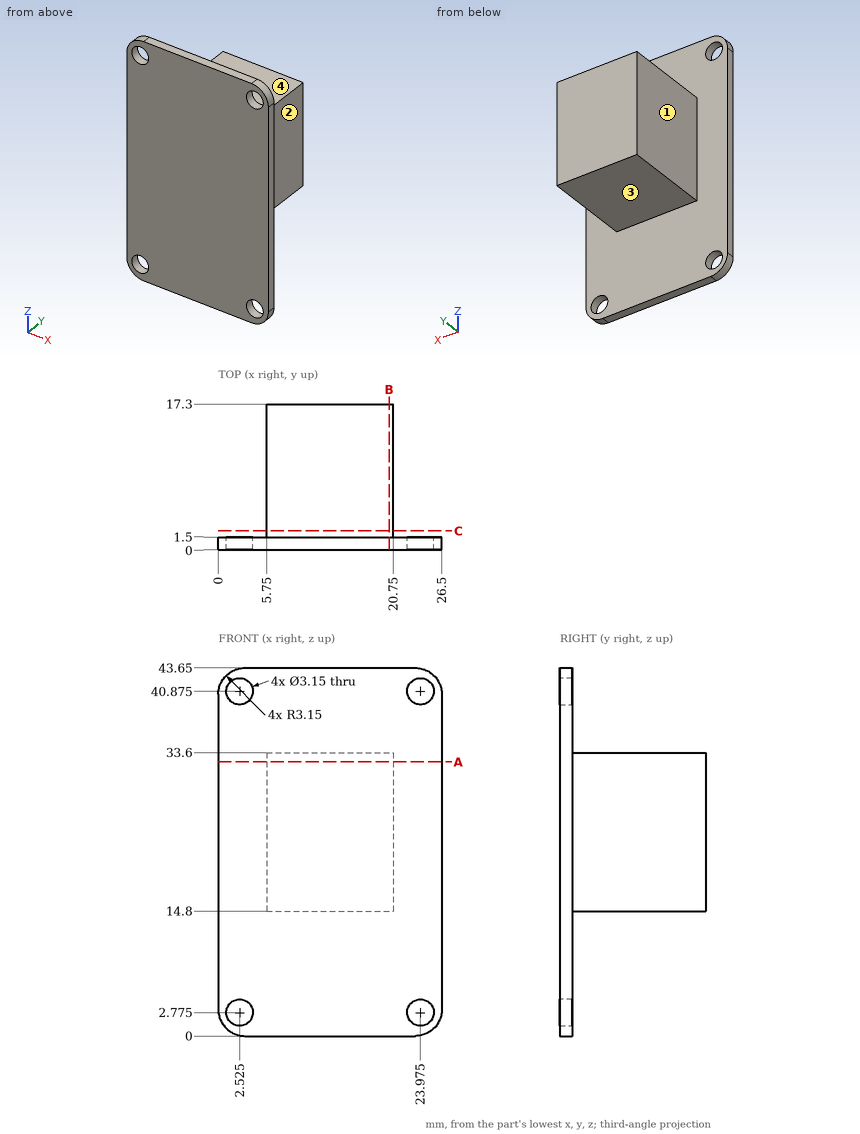
Check sheet for the drawn part. Datum: minimum x, y, z corner. Units: mm. A direction names the side the tool comes from. Coordinates: 2 decimals unless noted, no trailing zeros. Order: outer loops, then holes, each group sorted by start corner. A loop starts at its lowest first (then second) coordinate and runs counter-clockwise, first axis right, second up. Notation, with made-up numbers: M -39.5,-20.75 L -0.5,-20.75 A30 cw -0.5,8.25 Z; hole C -20,27 d6. An arc over 180 degrees is marked long. One line per question, with ' | ' between items. Start each with the question number.
Item 1: Material ranges on L1, parallel to Y at x = 21, z = 19.5; L2, parallel to X at y = 3.75, z = 26; L3, parallel to Z at x = 17, y = 13.5, recorded low to high. Write a range as [from, to].
Item 2: Set-up check for the marked faces 1, 2, 3 and 4: record each of +Z, -Z, +X, -X, +Y, -Y from which the full face is reachable in a straight line by a thin tool's end or side.
Item 3: Cross-section at B-B on x = 20.25. Enter the section's corners in (y, z), then the cut area to 3 significant figures.
Item 4: Cross-section at A-A on z = 32.5. Enter the section's corners in (x, y), then the cut area to 3 significant figures.
Item 5: Cross-section at C-C on y = 2.25. Enter the section's corners in (x, z), then the cut area to 3 significant figures.
Item 6: Gauge pin test, flat ends, axial feed: pin 1 (1.5 mm diameter, centred on x = 8, y = 4, fed in from +Z); pin 2 (2 mm diameter, centred on x = 10, y = 13, fed in from -Z); pin 3 (4 mm diameter, centred on x = 23.975, z = 40.875, fed in from +Y). Record the tip position at first contact, or that the pin passes through.
Findings:
1) L1: y = [0, 1.5] | L2: x = [5.75, 20.75] | L3: z = [14.8, 33.6]
2) face 1: +Z, -Z, -X, +Y | face 2: +Z, -Z, +X, +Y | face 3: -Z, +X, -X, +Y | face 4: +Z, +X, -X, +Y
3) outline: M 0,0 L 1.5,0 L 1.5,14.8 L 17.3,14.8 L 17.3,33.6 L 1.5,33.6 L 1.5,43.65 L 0,43.65 Z | area: 363 mm²
4) outline: M 0,0 L 26.5,0 L 26.5,1.5 L 20.75,1.5 L 20.75,17.3 L 5.75,17.3 L 5.75,1.5 L 0,1.5 Z | area: 277 mm²
5) outline: M 5.75,14.8 L 20.75,14.8 L 20.75,33.6 L 5.75,33.6 Z | area: 282 mm²
6) pin 1: stops at z = 33.6 | pin 2: stops at z = 14.8 | pin 3: stops at y = 1.5
